from build123d import *

# Parameters (mm, degrees)
SKETCH1_W               = 103.1875
SKETCH1_H               = 103.1875
SKETCH1_W_2             = 96.8375
SKETCH1_H_2             = 96.8375
BOSS_EXTRUDE1_DEPTH     = 266.7
SKETCH2_W               = 52.3875
SKETCH2_H               = 215.9
CUT_EXTRUDE2_DEPTH      = 52.59375
CUT_EXTRUDE2_DEPTH_BACK = 52.59375
SKETCH3_W               = 52.3875
SKETCH3_H               = 215.9
CUT_EXTRUDE3_DEPTH      = 52.59375
CUT_EXTRUDE3_DEPTH_BACK = 52.59375


with BuildPart() as part:
    # Sketch1 → Boss-Extrude1 (new body)
    with BuildSketch(Plane(origin=(0, 0, 0), x_dir=(1, 0, 0), z_dir=(0, 1, 0))):
        Rectangle(SKETCH1_W, SKETCH1_H)
        Rectangle(SKETCH1_W_2, SKETCH1_H_2, mode=Mode.SUBTRACT)
    extrude(amount=BOSS_EXTRUDE1_DEPTH)

    # Sketch2 → Cut-Extrude2 (cut, two sides)
    with BuildSketch(Plane.XY) as cut_extrude2_sk:
        with Locations((0, 133.35)):
            Rectangle(SKETCH2_W, SKETCH2_H)
    extrude(amount=CUT_EXTRUDE2_DEPTH, mode=Mode.SUBTRACT)
    extrude(cut_extrude2_sk.sketch, amount=-CUT_EXTRUDE2_DEPTH_BACK, mode=Mode.SUBTRACT)

    # Sketch3 → Cut-Extrude3 (cut, two sides)
    with BuildSketch(Plane(origin=(0, 0, 0), x_dir=(0, 0, -1), z_dir=(1, 0, 0))) as cut_extrude3_sk:
        with Locations((0, 133.35)):
            Rectangle(SKETCH3_W, SKETCH3_H)
    extrude(amount=CUT_EXTRUDE3_DEPTH, mode=Mode.SUBTRACT)
    extrude(cut_extrude3_sk.sketch, amount=-CUT_EXTRUDE3_DEPTH_BACK, mode=Mode.SUBTRACT)


solid = part.part
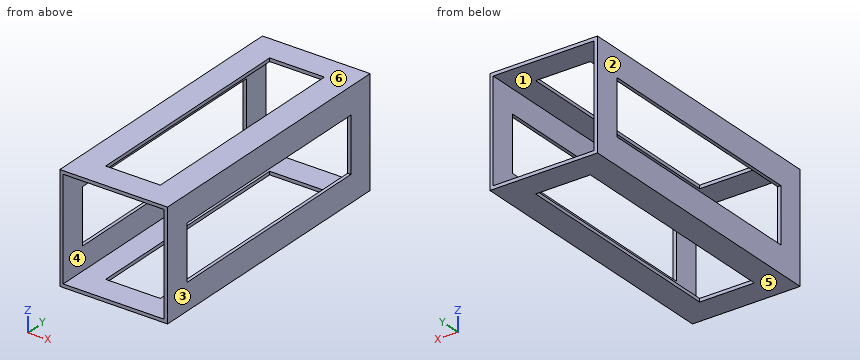
Read the model definition and answer for the solid it produces. Units are mm, in the model's axes. Face numbers are marked on the shaded views. A direction names the side the tool comes from. Round coordinates to 2 decimals unless told otherwise and drop trailing zeros. Write each loop counter-clockwise with the first axis right and the second up, starting at its lowest first coordinate (ties: lowest second). Pieces come first, ordered by that corner, then holes. Notation, with made-up numbers: (68, 12) - (119, 12) arc R18 cw to (119, 26) - close; hole circle Ø11 at (33, -21.5). An arc over 180 degrees is marked (long way). One line per question, with ' | ' between items. Start each with the question number.
1. Section C-C (z = -10.5) is taken. Determine the outline of the cut face in (x, y).
2. For the marked faces 1 and 2, determine the directions among +Z, -Z, +X, -X, +Y, -Y from which every point of the face is accessible in a straight line to the end or side of a thin tool.
3. Section D-D (x = 42.5) is taken. Determine the outline of the cut face in (y, z).
4. Find the intervals of material crossed by probe 1 along X at (y, z) = (17, 2), in increasing order. Write a range as [from, to].
5. Section B-B (x = -5) is taken. Determine the outline of the cut face in (y, z), and give its area (3 significant figures).
6. Section A-A (y = 153) is taken. Determine the outline of the cut face in (x, z), and give its area (3 significant figures).
7. For a pull along Z with two mould halves and no side action, classify the marked faces 3, 4, 5 and 6 as +Z half, -Z half, draft (parallel to the pull), parting line (faces both ways), or undercut.
8. This flat-tipped pin is pushed along its axis until it touches: pin 1 (6 mm diameter, centred on y = 44, z = -21.5, fed in from +X). Where does it stop, or does it pass through?
Filled in:
1) outline: (-51.59, 0) - (-48.42, 0) - (-48.42, 25.4) - (-51.59, 25.4) - close; (-51.59, 241.3) - (-48.42, 241.3) - (-48.42, 266.7) - (-51.59, 266.7) - close; (48.42, 0) - (51.59, 0) - (51.59, 25.4) - (48.42, 25.4) - close; (48.42, 241.3) - (51.59, 241.3) - (51.59, 266.7) - (48.42, 266.7) - close
2) face 1: +Y, -Y | face 2: +Z, -Z, -X, +Y, -Y
3) outline: (0, -51.59) - (266.7, -51.59) - (266.7, -48.42) - (0, -48.42) - close; (0, 48.42) - (266.7, 48.42) - (266.7, 51.59) - (0, 51.59) - close
4) probe 1: [-51.59, -48.42], [48.42, 51.59]
5) outline: (0, -51.59) - (25.4, -51.59) - (25.4, -48.42) - (0, -48.42) - close; (0, 48.42) - (25.4, 48.42) - (25.4, 51.59) - (0, 51.59) - close; (241.3, -51.59) - (266.7, -51.59) - (266.7, -48.42) - (241.3, -48.42) - close; (241.3, 48.42) - (266.7, 48.42) - (266.7, 51.59) - (241.3, 51.59) - close | area: 323 mm²
6) outline: (-51.59, -51.59) - (-26.19, -51.59) - (-26.19, -48.42) - (-48.42, -48.42) - (-48.42, -26.19) - (-51.59, -26.19) - close; (-51.59, 26.19) - (-48.42, 26.19) - (-48.42, 48.42) - (-26.19, 48.42) - (-26.19, 51.59) - (-51.59, 51.59) - close; (26.19, -51.59) - (51.59, -51.59) - (51.59, -26.19) - (48.42, -26.19) - (48.42, -48.42) - (26.19, -48.42) - close; (26.19, 48.42) - (48.42, 48.42) - (48.42, 26.19) - (51.59, 26.19) - (51.59, 51.59) - (26.19, 51.59) - close | area: 605 mm²
7) face 3: draft | face 4: undercut | face 5: -Z half | face 6: +Z half
8) pin 1: through
